Here's how the part is built. I have some questions about the finished solid (model axes, mm). Coordinates: 2 decimals unless noted, no trailing zeros. Write each loop counter-clockwise with the first axis right and the second up, starting at its lowest first coordinate (ties: lowest second). Pieces come first, ordered by that corner, then holes.
```python
from build123d import *

# Parameters (mm, degrees)
SKETCH1_W            = 142.875
SKETCH1_H            = 238.125
BOSS_EXTRUDE1_DEPTH  = 3
CUT_EXTRUDE1_START   = -3
CUT_EXTRUDE1_DEPTH   = 3
M5_CLEARANCE_HOLE1_D = 5.3
SKETCH5_R            = 9.779
SKETCH5_R_2          = 2.55
CUT_EXTRUDE2_DEPTH   = 139.881947396
FILLET1_R            = 6.35


# Read off the part's stored shape, not the designer's step: Cut-Extrude1
with BuildPart() as part:
    # Sketch1 → Boss-Extrude1 (new body)
    with BuildSketch(Plane(origin=(0, 0, 0), x_dir=(1, 0, 0), z_dir=(0, 1, 0))):
        Rectangle(SKETCH1_W, SKETCH1_H)
    extrude(amount=BOSS_EXTRUDE1_DEPTH)

    # Cut-Extrude1 outline → Cut-Extrude1 (cut)
    with BuildSketch(Plane(origin=(0, 3, 0), x_dir=(1, 0, 0), z_dir=(0, 1, 0)).offset(CUT_EXTRUDE1_START)):
        with BuildLine():
            ThreePointArc((71.4375, -116.313944107), (69.11044358, -117.711497264), (66.756056607, -119.0625))
            Line((66.756056607, -119.0625), (71.4375, -119.0625))
            Line((71.4375, -119.0625), (71.4375, -116.313944107))
        make_face()
        with BuildLine():
            Line((-71.4375, -119.0625), (-66.756056607, -119.0625))
            ThreePointArc((-66.756056607, -119.0625), (-69.11044358, -117.711497264), (-71.4375, -116.313944107))
            Line((-71.4375, -116.313944107), (-71.4375, -119.0625))
        make_face()
        with BuildLine():
            ThreePointArc((66.756056607, 119.0625), (69.11044358, 117.711497264), (71.4375, 116.313944107))
            Line((71.4375, 116.313944107), (71.4375, 119.0625))
            Line((71.4375, 119.0625), (66.756056607, 119.0625))
        make_face()
        with BuildLine():
            Line((-71.4375, 119.0625), (-71.4375, 116.313944107))
            ThreePointArc((-71.4375, 116.313944107), (-69.11044358, 117.711497264), (-66.756056607, 119.0625))
            Line((-66.756056607, 119.0625), (-71.4375, 119.0625))
        make_face()
    extrude(amount=CUT_EXTRUDE1_DEPTH, mode=Mode.SUBTRACT)

    # M5 Clearance Hole1 (through all)
    with Locations(Plane(origin=(0, 3, 0), x_dir=(1, 0, 0), z_dir=(0, 1, 0))):
        with Locations((65.0875, 0), (-65.0875, 112.7125), (65.0875, 112.7125), (65.0875, -112.7125), (-65.0875, -112.7125), (-65.0875, 0)):
            Hole(M5_CLEARANCE_HOLE1_D / 2)

    # Sketch5 → Cut-Extrude2 (cut, through all)
    with BuildSketch(Plane(origin=(0, 3, 0), x_dir=(1, 0, 0), z_dir=(0, 1, 0))):
        with Locations(Location((0, 0, 0), (0, 0, 270))):
            Circle(SKETCH5_R)
        with Locations(Location((-15, 15, 0), (0, 0, 270))):
            Circle(SKETCH5_R_2)
        with Locations(Location((15, 15, 0), (0, 0, 270))):
            Circle(SKETCH5_R_2)
        with Locations(Location((15, -15, 0), (0, 0, 270))):
            Circle(SKETCH5_R_2)
        with Locations(Location((-15, -15, 0), (0, 0, 270))):
            Circle(SKETCH5_R_2)
    extrude(amount=-CUT_EXTRUDE2_DEPTH, mode=Mode.SUBTRACT)

    # Fillet1
    fillet1_edges = [part.edges().sort_by_distance(p)[0] for p in [
        (71.4375, 1.5, 116.313944107),
        (71.4375, 1.5, -116.313944107),
        (66.756056607, 1.5, -119.0625),
        (-66.756056607, 1.5, -119.0625),
        (-71.4375, 1.5, -116.313944107),
        (-71.4375, 1.5, 116.313944107),
        (-66.756056607, 1.5, 119.0625),
        (66.756056607, 1.5, 119.0625),
    ]]
    fillet(fillet1_edges, radius=FILLET1_R)


solid = part.part
```
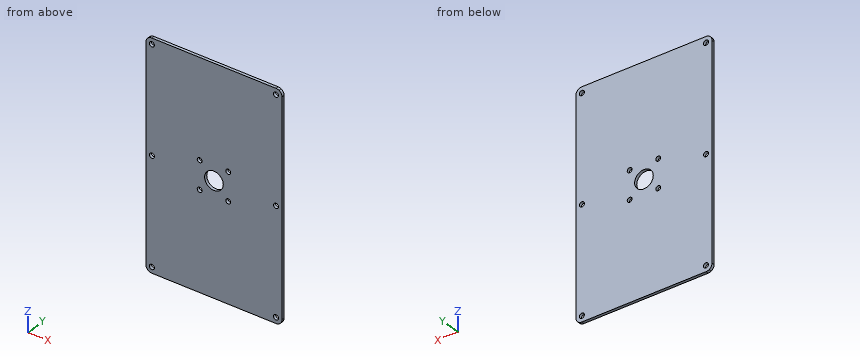
1) Imagine slicing it at D-D on y = 2.45. Count the separate pieces of the cut face and the enclosed holes in it, then the cut area to 3 significant figures.
Values follow:
separate pieces: 1
enclosed holes: 11
area: 33,500 mm2
2) Imagine slicing it at B-B on x = 0. Please give me the cut outline in (y, z), then the cut area to 3 significant figures.
Values follow:
outline: (0, -119.06) - (3, -119.06) - (3, -9.78) - (0, -9.78) - close; (0, 9.78) - (3, 9.78) - (3, 119.06) - (0, 119.06) - close
area: 656 mm2
3) Imagine slicing it at C-C on x = 15. Please give me the cut outline in (y, z).
Values follow:
outline: (0, -119.06) - (3, -119.06) - (3, -17.55) - (0, -17.55) - close; (0, -12.45) - (3, -12.45) - (3, 12.45) - (0, 12.45) - close; (0, 17.55) - (3, 17.55) - (3, 119.06) - (0, 119.06) - close
4) Imagine slicing it at A-A on z = 0. Please give me the cut outline in (x, y).
Values follow:
outline: (-71.44, 0) - (-67.74, 0) - (-67.74, 3) - (-71.44, 3) - close; (-62.44, 0) - (-9.78, 0) - (-9.78, 3) - (-62.44, 3) - close; (9.78, 0) - (62.44, 0) - (62.44, 3) - (9.78, 3) - close; (67.74, 0) - (71.44, 0) - (71.44, 3) - (67.74, 3) - close
5) I need wall thicknesses on probe 1 along X at (y, z) = (1, 15); probe 2 along Z at (x, y) = (-63, 0.6); probe 3 along Z at (x, y) = (16, 0.45). Which ranges of each line are inside material? Lowest first, please.
Values follow:
probe 1: x = -71.44 to -17.55, -12.45 to 12.45, 17.55 to 71.44
probe 2: z = -119.06 to -114.34, -111.08 to -1.63, 1.63 to 111.08, 114.34 to 119.06
probe 3: z = -119.06 to -17.35, -12.65 to 12.65, 17.35 to 119.06
